Answer from the drawing. Dimensions are ordinates in mm from the lowest x, y and z of the part. A direction names the side the tool comes from. Give positions to 0.01 mm unless a question says otherwise; leave off trailing zeros. Order: outer loops, then holes, each group sorted by start corner. A loop starts at its lowest first (then second) coordinate and runs counter-clockwise, first axis right, second up. Notation, with made-up numbers: (81.25, 80.25) - (108.25, 80.25) arc R12 ccw to (108.25, 91.25) - close; hole circle Ø2 at (14.25, -31). An arc over 180 degrees is marked (long way). Write each question's results on one line, items separated by ' | '.
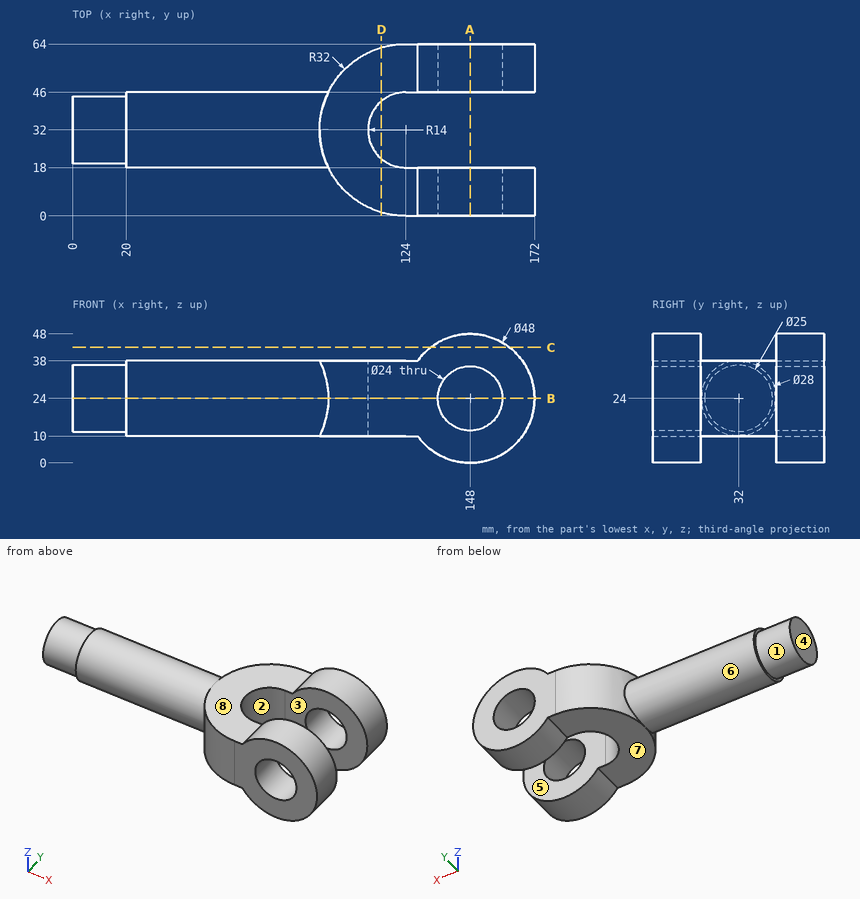
1. A cutting plane is placed at A-A, the plane x = 148. Write down the section's boundary in (y, z), then the cut area to 3 significant figures.
Answer list:
outline: (0, 0) - (18, 0) - (18, 12) - (0, 12) - close; (0, 36) - (18, 36) - (18, 48) - (0, 48) - close; (46, 0) - (64, 0) - (64, 12) - (46, 12) - close; (46, 36) - (64, 36) - (64, 48) - (46, 48) - close | area: 864 mm^2
2. Determine the mould class of the marked faces 1, 2, 3 and 4 for opening direction Y: +Y half, -Y half, draft (parallel to the pull), parting line (faces both ways), or undercut.
Answer list:
face 1: parting line | face 2: undercut | face 3: undercut | face 4: draft
3. A cutting plane is placed at C-C, the plane z = 43. Write down the section's boundary in (x, y), then the cut area to 3 significant figures.
Answer list:
outline: (133.34, 0) - (162.66, 0) - (162.66, 18) - (133.34, 18) - close; (133.34, 46) - (162.66, 46) - (162.66, 64) - (133.34, 64) - close | area: 1,060 mm^2
4. A tool of negligible diameter and unlimited length cuts with its end or side. For the marked faces 5, 6, 7 and 8, from which of +Z, -Z, +X, -X, +Y, -Y can it reach the whole face along a straight path? Write none if from no direction.
Answer list:
face 5: +Z, -Z, +X | face 6: -X | face 7: -Z, -X, +Y, -Y | face 8: +Z, -X, +Y, -Y
5. Given P1, Ø14.5, axis at x = 149.5, z = 28, coming from the +Y side; P2, Ø5, axis at x = 70.5, z = 10.5, coming from the +Y side; P3, Ø2, axis at x = 39.5, y = 40, coming from the -Z side; P4, Ø1, axis at x = 22.5, z = 15.5, coming from the -Y side, each flat-ended and moving along its own axis, determine where each tip first touches the part or whether it passes through.
Answer list:
P1: through | P2: y = 40.66 | P3: z = 11.88 | P4: y = 20.51
6. A cutting plane is placed at B-B, the plane z = 24. Write down the section's boundary in (x, y).
Answer list:
outline: (0, 19.5) - (20, 19.5) - (20, 18) - (95.23, 18) arc R32 ccw to (124, 0) - (136, 0) - (136, 18) - (124, 18) arc R14 cw to (124, 46) - (136, 46) - (136, 64) - (124, 64) arc R32 ccw to (95.23, 46) - (20, 46) - (20, 44.5) - (0, 44.5) - close; (160, 0) - (172, 0) - (172, 18) - (160, 18) - close; (160, 46) - (172, 46) - (172, 64) - (160, 64) - close
7. Straight lines are drawn through the part: line 1 (X direction, y = 4.5, z = 24); line 2 (Z direction, x = 70.5, y = 32.5); line 3 (X direction, y = 23, z = 15). For each, find the intervals that lie inside material, in ascending order. Write a range as [from, to].
Answer list:
line 1: [107.64, 136], [160, 172] | line 2: [10.01, 37.99] | line 3: [20, 113.28]
8. A cutting plane is placed at D-D, the plane x = 115. Write down the section's boundary in (y, z).
Answer list:
outline: (1.29, 10) - (21.28, 10) - (21.28, 38) - (1.29, 38) - close; (42.72, 10) - (62.71, 10) - (62.71, 38) - (42.72, 38) - close
